```python
from build123d import *

# Parameters (mm, degrees)
F0_W     = 152.3854583502
F0_H     = 152.996212244
F1_DEPTH = 254
F2_W     = 152.3854583502
F2_H     = 254
F3_DEPTH = 25.4
F4_T     = -2.54


with BuildPart() as f1:
    # F0 (on Front) → F1 (new body)
    with BuildSketch(Plane.XZ):
        Rectangle(F0_W, F0_H)
    extrude(amount=F1_DEPTH)

    # F2 (on face) → F3 (cut)
    with BuildSketch(Plane.XY.offset(76.498106122)):
        with Locations((0, -127)):
            Rectangle(F2_W, F2_H)
    extrude(amount=-F3_DEPTH, mode=Mode.SUBTRACT)

    # F4
    f4_openings = [f1.faces().sort_by_distance(p)[0] for p in [
        (0, -127, 51.098106),
    ]]
    offset(amount=F4_T, openings=f4_openings)


solid = f1.part
```
Work out the finished part from the listing and answer in its coordinate system (mm). A direction names the side the tool comes from. Round coordinates to 2 decimals unless told otherwise and drop trailing zeros. Order: outer loops, then holes, each group sorted by start corner. A loop starts at its lowest first (then second) coordinate and runs counter-clockwise, first axis right, second up.
Q1. A cutting plane is placed at C-C, the plane y = -123.5. Determine the outline of the cut face in (x, z), then the cut area to 3 significant figures.
Solution:
outline: (-76.19, -76.5) - (76.19, -76.5) - (76.19, 51.1) - (73.65, 51.1) - (73.65, -73.96) - (-73.65, -73.96) - (-73.65, 51.1) - (-76.19, 51.1) - close
area: 1,020 mm2
Q2. A cutting plane is placed at A-A, the plane z = 5.5. Determine the outline of the cut face in (x, y), then the cut area to 3 significant figures.
Solution:
outline: (-76.19, -254) - (76.19, -254) - (76.19, 0) - (-76.19, 0) - close; hole (-73.65, -251.46) - (73.65, -251.46) - (73.65, -2.54) - (-73.65, -2.54) - close
area: 2,040 mm2
Q3. Find the intervals of material crossed by line 1 along Y through (x, z) = (-61, 22); line 2 along X through (y, z) = (-82, 19); line 3 along Z through (x, y) = (8.5, -129), in increasing order.
Solution:
line 1: y = -254 to -251.46, -2.54 to 0
line 2: x = -76.19 to -73.65, 73.65 to 76.19
line 3: z = -76.5 to -73.96
Q4. A cutting plane is placed at B-B, the plane x = 49.5. Determine the outline of the cut face in (y, z).
Solution:
outline: (-254, -76.5) - (0, -76.5) - (0, 51.1) - (-2.54, 51.1) - (-2.54, -73.96) - (-251.46, -73.96) - (-251.46, 51.1) - (-254, 51.1) - close
Q5. A tool of negligible diameter and unlimited length cuts with its end or side. For faces 4 (the flat face through (-1, -125, -76.498)), 5 (the flat face through (-1, -2.54, -11)), from which of +Z, -Z, +X, -X, +Y, -Y can it reach the whole face along a straight path? Write none if from no direction.
Solution:
face 4: -Z, +X, -X, +Y, -Y
face 5: +Z
Q6. The mould has two halves that part along X. Classify faces 1 (the flat face through (-1, -254, -12)), 2 (the flat face through (-1, -125, -73.958)), 3 (the flat face through (76.193, -125, -14)): pulls with the +X half, pulls with the -X half, needs draft (parallel to the pull), parting line crosses it, or undercut.
Solution:
face 1: needs draft
face 2: undercut
face 3: pulls with the +X half
